```python
from build123d import *

# Parameters (mm, degrees)
F0_W     = 81.788
F0_H     = 168.402
F1_DEPTH = 64.77
F2_W     = 76.708
F2_H     = 163.322
F3_DEPTH = 62.23
F5_DEPTH = 81.788
F7_DEPTH = 177.8


with BuildPart() as f1:
    # F0 (on Top) → F1 (new body)
    with BuildSketch(Plane.XY):
        Rectangle(F0_W, F0_H)
    extrude(amount=F1_DEPTH)

    # F2 (on face) → F3 (cut)
    with BuildSketch(Plane.XY.offset(64.77)):
        Rectangle(F2_W, F2_H)
    extrude(amount=-F3_DEPTH, mode=Mode.SUBTRACT)

    # F4 (on face) → F5 (join)
    with BuildSketch(Plane.YZ.offset(40.894)):
        Polygon((26.035, 64.77), (66.175841, 0), (68.715841, 0), (28.575, 64.77), align=None)
        Polygon((10.287, 64.77), (50.427841, 0), (52.967841, 0), (12.827, 64.77), align=None)
        Polygon((-5.461, 64.77), (34.679841, 0), (37.219841, 0), (-2.921, 64.77), align=None)
        Polygon((-21.209, 64.77), (18.931841, 0), (21.471841, 0), (-18.669, 64.77), align=None)
        Polygon((-36.957, 64.77), (3.183841, 0), (5.723841, 0), (-34.417, 64.77), align=None)
        Polygon((-52.705, 64.77), (-12.564159, 0), (-10.024159, 0), (-50.165, 64.77), align=None)
        Polygon((-68.453, 64.77), (-28.312159, 0), (-25.772159, 0), (-65.913, 64.77), align=None)
    extrude(amount=-F5_DEPTH)

    # F6 (on face) → F7 (cut)
    with BuildSketch(Plane.XZ.offset(84.201)):
        with BuildLine():
            Line((28.829, 64.77), (-28.829, 64.77))
            ThreePointArc((-28.829, 64.77), (0, 40.450578), (28.829, 64.77))
        make_face()
    extrude(amount=-F7_DEPTH, mode=Mode.SUBTRACT)


solid = f1.part
```
Verification items for the finished model (mm, model axes). A direction names the side the tool comes from. Coordinates: 2 decimals unless noted, no trailing zeros. Write each loop counter-clockwise with the first axis right and the second up, starting at its lowest first coordinate (ties: lowest second). Pieces come first, ordered by that corner, then holes. Notation, with made-up numbers: M 40,-18.75 L 76,-18.75 A15 ccw 76,7.25 Z; hole C 73.5,25.25 d9. An arc over 180 degrees is marked long. Answer as a JSON object with one key per item and string values. Group by question number.
(1) Cross-section at B-B, the plane z = 12. State how many separate pieces and enclosed holes the cut face has, and give its area (3 significant figures).
(2) Cross-section at A-A, the plane y = 56.5. Record the cut outline in (x, z), and give its area (3 significant figures).
(3) Tool access check on faces 4 (the face through (40.894, -1, 33)), 5 (the face through (-38.354, 23, 34)), 6 (the face through (-1, 75, 2.54)). Record the directions out of +Z, -Z, +X, -X, +Y, -Y that give a thin tool (end or side, any length) a straight path to the whole face; none if there is none.
(4) Material ranges on line 1 (X direction, y = 46, z = 44); line 2 (Z direction, x = 36.5, y = -38.5); line 3 (Z direction, x = 24.5, y = -16.5), recorded low to high.
(5) Gauge pin test, flat ends, axial feed: pin 1 (6.5 mm diameter, centred on x = -13, y = 28, fed in from +Z); pin 2 (10.5 mm diameter, centred on x = 10, y = 44, fed in from +Z); pin 3 (14.5 mm diameter, centred on x = -15, y = 11, fed in from +Z). Record the tip position at first contact, or that the pin passes through.
(6) Cross-section at C-C, the plane y = -40. Record the cut outline in (x, z), and give its area (3 significant figures).
(7) Release check for a two-part mould opening along Z. For faces 1 (the face through (0.537, 17.838, 27.176)), 2 (the face through (-0.19, -37.42, 40.45)), 3 (the face through (-1, 81.661, 27)) record: +Z half, -Z half, draft (parallel to the pull), parting line (faces both ways), or undercut.
Reply:
{
 "1": {"separate pieces": "1", "enclosed holes": "8", "area": "2,610 mm²"},
 "2": {"outline": "M -40.89,0 L 40.89,0 L 40.89,64.77 L 38.35,64.77 L 38.35,19.71 L -38.35,19.71 L -38.35,64.77 L -40.89,64.77 Z; hole M -38.35,2.54 L 38.35,2.54 L 38.35,15.61 L -38.35,15.61 Z", "area": "838 mm²"},
 "3": {"face 4": "+Z, -Z, +X, +Y, -Y", "face 5": "none", "face 6": "+Z"},
 "4": {"line 1": "-40.89 to -38.35, 38.35 to 40.89", "line 2": "0 to 2.54, 16.44 to 20.54, 41.85 to 45.95", "line 3": "0 to 2.54, 6.35 to 10.45, 31.76 to 35.86"},
 "5": {"pin 1": "z = 44.53", "pin 2": "z = 44.29", "pin 3": "z = 49.2"},
 "6": {"outline": "M -40.89,0 L 40.89,0 L 40.89,64.77 L 38.35,64.77 L 38.35,48.37 L 20.01,48.37 A29.25 cw 14.45,44.27 L 38.35,44.27 L 38.35,22.96 L -38.35,22.96 L -38.35,44.27 L -14.45,44.27 A29.25 cw -20.01,48.37 L -38.35,48.37 L -38.35,64.77 L -40.89,64.77 Z; hole M -38.35,2.54 L 38.35,2.54 L 38.35,18.86 L -38.35,18.86 Z", "area": "1,010 mm²"},
 "7": {"face 1": "undercut", "face 2": "+Z half", "face 3": "draft"}
}
